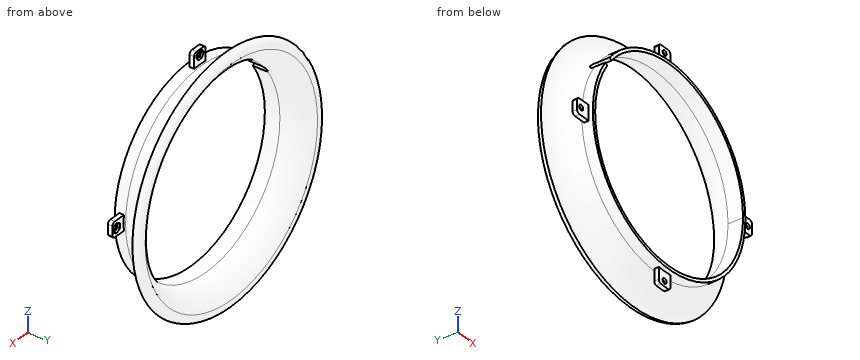
```python
from build123d import *

# Parameters (mm, degrees)
BOSS_EXTRUDE1_DEPTH = 3
SKETCH5_R           = 1.7
CUT_EXTRUDE2_DEPTH  = 7
CUT_EXTRUDE1_DEPTH  = 1.5
CIRPATTERN13_COUNT  = 4
CUT_EXTRUDE3_DEPTH  = 113.339059349


with BuildPart() as part:
    # Sketch1 → Revolve1 (revolve)
    with BuildSketch(Plane.XY):
        with BuildLine():
            Line((63.75, 18.737026277), (63.75, 25.098484685))
            ThreePointArc((63.75, 25.098484685), (66.610296039, 35.058746011), (74.319544881, 41.983742863))
            ThreePointArc((74.319544881, 41.983742863), (78.398172265, 41.784089154), (80.425886783, 38.239595286))
            ThreePointArc((80.425886783, 38.239595286), (69.983309328, 33.20133547), (65.75, 22.407328891))
            Line((65.75, 22.407328891), (65.75, 18.737026277))
            Line((65.75, 18.737026277), (65.75, 15.098484685))
            Line((65.75, 15.098484685), (63.75, 15.098484685))
            Line((63.75, 15.098484685), (63.75, 18.737026277))
        make_face()
    revolve(axis=Axis((0, 0, 0), (0, 1, 0)))

    # Sketch3 → Boss-Extrude1 (add)
    with BuildSketch(Plane(origin=(0, 18.098484685, 0), x_dir=(-1, 0, 0), z_dir=(0, -1, 0))):
        with BuildLine():
            Line((65.55961028, 5), (73.36961028, 5))
            ThreePointArc((73.36961028, 5), (74.783823842, 4.414213562), (75.36961028, 3))
            Line((75.36961028, 3), (75.36961028, -3))
            ThreePointArc((75.36961028, -3), (74.783823842, -4.414213562), (73.36961028, -5))
            Line((73.36961028, -5), (65.55961028, -5))
            ThreePointArc((65.55961028, -5), (65.75, 0), (65.55961028, 5))
        make_face()
    boss_extrude1 = extrude(amount=-BOSS_EXTRUDE1_DEPTH)

    # Sketch5 → Cut-Extrude2 (cut, through all)
    with BuildSketch(Plane(origin=(0, 21.098484685, 0), x_dir=(1, 0, 0), z_dir=(0, 1, 0))):
        with Locations((-71.86961028, 0)):
            Circle(SKETCH5_R)
    cut_extrude2 = extrude(amount=-CUT_EXTRUDE2_DEPTH, mode=Mode.SUBTRACT)

    # Sketch4 → Cut-Extrude1 (cut)
    with BuildSketch(Plane(origin=(0, 21.098484685, 0), x_dir=(1, 0, 0), z_dir=(0, 1, 0))):
        Polygon((-71.86961028, 3.290896534), (-74.71961028, 1.645448267), (-74.71961028, -1.645448267), (-71.86961028, -3.290896534), (-69.01961028, -1.645448267), (-69.01961028, 1.645448267), align=None)
    cut_extrude1 = extrude(amount=-CUT_EXTRUDE1_DEPTH, mode=Mode.SUBTRACT)

    # CirPattern13: Boss-Extrude1, Cut-Extrude2, Cut-Extrude1 ×4 about axis
    cirpattern13_axis = Axis((0, 0, 0), (0, 1, 0))
    for i in range(1, CIRPATTERN13_COUNT):
        add(boss_extrude1.rotate(cirpattern13_axis, i * 360 / CIRPATTERN13_COUNT))
        add(cut_extrude2.rotate(cirpattern13_axis, i * 360 / CIRPATTERN13_COUNT), mode=Mode.SUBTRACT)
        add(cut_extrude1.rotate(cirpattern13_axis, i * 360 / CIRPATTERN13_COUNT), mode=Mode.SUBTRACT)

    # Sketch6 → Cut-Extrude3 (cut, through all)
    with BuildSketch(Plane(origin=(0, 0, 0), x_dir=(0, 1, 0), z_dir=(0.809016994, 0, -0.587785252))):
        with BuildLine():
            Line((21, 3.175), (15.098484685, 3.175))
            Line((15.098484685, 3.175), (15.098484685, -3.175))
            Line((15.098484685, -3.175), (21, -3.175))
            Line((21, -3.175), (23, -3.175))
            ThreePointArc((23, -3.175), (26.175, 0), (23, 3.175))
            Line((23, 3.175), (21, 3.175))
        make_face()
    extrude(amount=-CUT_EXTRUDE3_DEPTH, mode=Mode.SUBTRACT)


solid = part.part
```
Part model, mm, in its own coordinate system. Round coordinates to 2 decimals unless told otherwise and drop trailing zeros. Order: outer loops, then holes, each group sorted by start corner. A loop starts at its lowest first (then second) coordinate and runs counter-clockwise, first axis right, second up. Notation, with made-up numbers: M -11,8.25 L -5,8.25 A18 cw -5,22.25 Z; hole C -26.5,12 d11. An arc over 180 degrees is marked long. Put each result on its own line as item: value. Start each with the question number.
1. Drill centre lines: probe 1 along X at (y, z) = (20.25, 66); probe 2 along Z at (x, y) = (32.5, 36.5); probe 3 along Z at (x, y) = (43, 35). Where is each one in solid material? Low to high. Write a range as [from, to].
2. Slice it at A-A on y = 32.75. List the corners of the cut face in (x, z), then the cut area to 3 significant figures.
3. Drop flat-ended pins along their axis: pin 1 (3 mm diameter, centred on x = -72, z = 1, fed in from +Y); pin 2 (4 mm diameter, centred on x = 0, z = -71.87, fed in from -Y); pin 3 (8 mm diameter, centred on x = 2, z = -70, fed in from +Y). Give the stop position or say it passes through.
Findings:
1. probe 1: [-5, 5]
1. probe 2: [-66.83, -59.29], [59.29, 66.83]
1. probe 3: [-57.7, -50.82], [50.82, 57.7]
2. outline: C 0,0 d139.16; hole C 0,0 d130.76
2. area: 1,780 mm2
3. pin 1: y = 41.56
3. pin 2: y = 18.1
3. pin 3: y = 41.84
